Check sheet for the modelled part. Datum: model origin and axes. Units: mm. A direction names the side the tool comes from. Give positions to 0.01 mm unless a question says otherwise; leave off trailing zeros. Order: outer loops, then holes, each group sorted by start corner. A loop starts at its lowest first (then second) coordinate and runs counter-clockwise, first axis right, second up.
Item 1: Access from +Z, -Z, +X, -X, +Y, -Y to the whole of each face (thin tool, end or side, straight path). Record for faces 5 (the cylindrical face through (16.05, 2.07, -9.03)), 6 (the flat face through (-27.864, 0.044, 5.455)), 7 (the flat face through (-9, -3.175, -1)).
Item 2: Sectioned sample at D-D on y = -2. Count the separate pieces of the cut face and the enclosed holes in it, and give its area (3 significant figures).
Item 3: Sectioned sample at A-A on x = 0. Record the boundary of the cut face in (y, z) (3 decimals), and give its area (3 significant figures).
Item 4: Gauge pin test, flat ends, axial feed: P1, Ø1.9, axis at y = -1.5, z = -27, coming from the +X side; P2, Ø1.5, axis at x = 10, y = 2, coming from the -Z side; P3, Ø11, axis at x = 3.5, z = -4, coming from the +Y side. Record the tip position at first contact, or that the pin passes through.
Item 5: Sectioned sample at C-C on x = -31.5. Record the boundary of the cut face in (y, z) (3 decimals).
Item 6: Sectioned sample at B-B on z = -24.5. Record the boundary of the cut face in (x, y) (1 decimal).
Item 7: Release check for a two-part mould opening along Z. For faces 1 (the flat face through (0, 0, -36.195)), 2 (the cylindrical face through (40.924, 0.044, -5.373)), 3 (the flat face through (19, 3.175, -1)), 4 (the flat face through (-15.333, -0.661, 9.002)) record: released by +Z, released by -Z, zero draft, split by the parting line, or undercut.
Item 8: Material ranges on line 1 along Z through (x, y) = (18, -2.25); line 2 along X through (y, z) = (1.25, 22.5); line 3 along Y through (x, z) = (-10, 7.5) (3 decimals), recorded low to high.
from build123d import *

# Parameters (mm, degrees)
SKETCH1_R           = 44.45
SKETCH1_R_2         = 6.35
BOSS_EXTRUDE1_DEPTH = 3.175
SKETCH5_W           = 18.415
SKETCH5_H           = 18.415
CUT_EXTRUDE4_DEPTH  = 64.181702256
CIRPATTERN2_COUNT   = 3
SKETCH3_R           = 44.45
SKETCH3_R_2         = 41.275
CUT_EXTRUDE2_DEPTH  = 64.181702256
SKETCH6_R           = 18.415
CUT_EXTRUDE5_DEPTH  = 2.2352
SKETCH7_R           = 2.4892
CUT_EXTRUDE6_DEPTH  = 59.716043378
CIRPATTERN3_COUNT   = 3


with BuildPart() as part:
    # Sketch1 → Boss-Extrude1 (new, symmetric)
    with BuildSketch(Plane(origin=(0, 0, 0), x_dir=(1, 0, 0), z_dir=(0, 1, 0))):
        with Locations(Location((0, 0, 0), (0, 0, 270))):
            Circle(SKETCH1_R)
        with Locations(Location((0, 0, 0), (0, 0, 270))):
            Circle(SKETCH1_R_2, mode=Mode.SUBTRACT)
    extrude(amount=BOSS_EXTRUDE1_DEPTH, both=True)

    # Sketch5 → Cut-Extrude4 (cut, through all)
    with BuildSketch(Plane(origin=(0, 3.175, 0), x_dir=(1, 0, 0), z_dir=(0, 1, 0))):
        with Locations((0, 26.9875)):
            Rectangle(SKETCH5_W, SKETCH5_H)
    cut_extrude4 = extrude(amount=-CUT_EXTRUDE4_DEPTH, mode=Mode.SUBTRACT)

    # CirPattern2: Cut-Extrude4 ×3 about axis
    cirpattern2_axis = Axis((0, 0, 0), (0, 1, 0))
    for i in range(1, CIRPATTERN2_COUNT):
        add(cut_extrude4.rotate(cirpattern2_axis, i * 360 / CIRPATTERN2_COUNT), mode=Mode.SUBTRACT)

    # Sketch3 → Cut-Extrude2 (cut, through all)
    with BuildSketch(Plane(origin=(0, 3.175, 0), x_dir=(1, 0, 0), z_dir=(0, 1, 0))):
        Circle(SKETCH3_R)
        with Locations(Location((0, 0, 0), (0, 0, 270))):
            Circle(SKETCH3_R_2, mode=Mode.SUBTRACT)
    extrude(amount=-CUT_EXTRUDE2_DEPTH, mode=Mode.SUBTRACT)

    # Sketch6 → Cut-Extrude5 (cut)
    with BuildSketch(Plane(origin=(0, 3.175, 0), x_dir=(1, 0, 0), z_dir=(0, 1, 0))):
        Circle(SKETCH6_R)
    extrude(amount=-CUT_EXTRUDE5_DEPTH, mode=Mode.SUBTRACT)

    # Sketch7 → Cut-Extrude6 (cut, through all)
    with BuildSketch(Plane(origin=(0, 3.175, 0), x_dir=(1, 0, 0), z_dir=(0, 1, 0))):
        with Locations(Location((-16.34406614, 16.34406614, 0), (0, 0, 270))):
            Circle(SKETCH7_R)
        with Locations(Location((-22.326409549, 5.982343408, 0), (0, 0, 270))):
            Circle(SKETCH7_R)
    cut_extrude6 = extrude(amount=-CUT_EXTRUDE6_DEPTH, mode=Mode.SUBTRACT)

    # CirPattern3: Cut-Extrude6 ×3 about axis
    cirpattern3_axis = Axis((0, 0, 0), (0, 1, 0))
    for i in range(1, CIRPATTERN3_COUNT):
        add(cut_extrude6.rotate(cirpattern3_axis, i * 360 / CIRPATTERN3_COUNT), mode=Mode.SUBTRACT)


solid = part.part
Report:
1. face 5: +Y
1. face 6: +Y, -Y
1. face 7: +Z, -Z, +X, -X, -Y
2. separate pieces: 1
2. enclosed holes: 10
2. area: 4,090 mm2
3. outline: (-3.175, -41.275) - (3.175, -41.275) - (3.175, -36.195) - (-3.175, -36.195) - close; (-3.175, -17.78) - (0.94, -17.78) - (0.94, -6.35) - (-3.175, -6.35) - close; (-3.175, 6.35) - (0.94, 6.35) - (0.94, 18.415) - (3.175, 18.415) - (3.175, 41.275) - (-3.175, 41.275) - close
3. area: 274 mm2
4. P1: stops at x = 32.02
4. P2: stops at z = -40.23
4. P3: stops at y = 0.94
5. outline: (-3.175, -26.672) - (3.175, -26.672) - (3.175, 7.555) - (-3.175, 7.555) - close; (-3.175, 17.83) - (3.175, 17.83) - (3.175, 26.672) - (-3.175, 26.672) - close
6. outline: (-33.2, -3.2) - (-9.2, -3.2) - (-9.2, 3.2) - (-33.2, 3.2) - close; (9.2, -3.2) - (33.2, -3.2) - (33.2, 3.2) - (9.2, 3.2) - close
7. face 1: undercut
7. face 2: split by the parting line
7. face 3: zero draft
7. face 4: undercut
8. line 1: z = -37.14 to -18.2, -14.49 to 4.38, 21.02 to 37.14
8. line 2: x = -34.6 to -28.8, -20.56 to -8.47, -3.5 to 3.5, 8.47 to 20.56, 28.8 to 34.6
8. line 3: y = -3.175 to 0.94
